Drawing for the job (mm, zero at the part's lowest x, y, z). A direction names the side the tool comes from. Give positions to 0.01 mm unless a question says otherwise; leave off trailing zeros. Write each loop counter-clockwise with the first axis right and the second up, starting at its lowest first coordinate (ties: lowest second). Pieces come first, ordered by that corner, then holes.
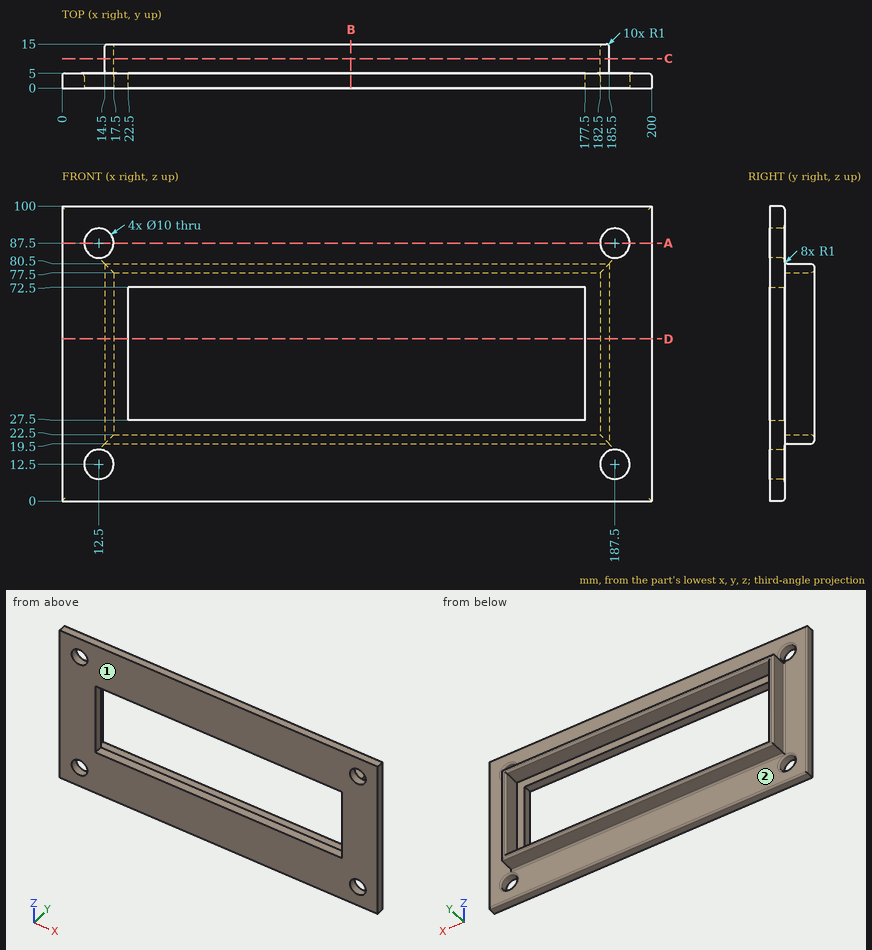
1. Which spindle directions (+Z, -Z, +X, -X, +Y, -Y) get a long thin tool onto all of the face, cutting with end or side? Do the marked faces 1 and 2. Say none if no direction does.
Calculated:
face 1: +Z, -Z, +X, -X, -Y
face 2: +Y
2. Slice it at D-D, the plane z = 55. Write the cut outline in (x, y), and give its area (3 significant figures).
Calculated:
outline: (0, 0) - (22.5, 0) - (22.5, 5) - (17.5, 5) - (17.5, 14) arc R1 ccw to (16.5, 15) - (15.5, 15) arc R1 ccw to (14.5, 14) - (14.5, 6) arc R1 cw to (13.5, 5) - (1, 5) arc R1 ccw to (0, 4) - close; (177.5, 0) - (200, 0) - (200, 4) arc R1 ccw to (199, 5) - (186.5, 5) arc R1 cw to (185.5, 6) - (185.5, 14) arc R1 ccw to (184.5, 15) - (183.5, 15) arc R1 ccw to (182.5, 14) - (182.5, 5) - (177.5, 5) - close
area: 284 mm2
3. Pin check, flat tips, straight feed: P1, Ø8, axis at x = 12.5, z = 12.5, coming from the -Y side; P2, Ø4, axis at x = 98, y = 10, coming from the -Z side; P3, Ø5, axis at x = 36, y = 13, coming from the +Z side; P4, Ø1, axis at y = 11.5, z = 44.5, coming from the -X side. Stop position of each tip, or through.
Calculated:
P1: passes through
P2: stops at z = 19.5
P3: stops at z = 80.5
P4: stops at x = 14.5
4. Probe probe 1 along X at (y, z) = (0.95, 12.5); probe 2 along X at (y, z) = (10, 34); probe 3 along Z at (x, y) = (24, 8.25). List the from-to ranges inside material, lowest first.
Calculated:
probe 1: x = 0 to 7.5, 17.5 to 182.5, 192.5 to 200
probe 2: x = 14.5 to 17.5, 182.5 to 185.5
probe 3: z = 19.5 to 22.5, 77.5 to 80.5
5. Slice it at B-B, the plane x = 98. Write the cut outline in (y, z).
Calculated:
outline: (0, 0) - (4, 0) arc R1 ccw to (5, 1) - (5, 18.5) arc R1 cw to (6, 19.5) - (14, 19.5) arc R1 ccw to (15, 20.5) - (15, 21.5) arc R1 ccw to (14, 22.5) - (5, 22.5) - (5, 27.5) - (0, 27.5) - close; (0, 72.5) - (5, 72.5) - (5, 77.5) - (14, 77.5) arc R1 ccw to (15, 78.5) - (15, 79.5) arc R1 ccw to (14, 80.5) - (6, 80.5) arc R1 cw to (5, 81.5) - (5, 99) arc R1 ccw to (4, 100) - (0, 100) - close
6. Slice it at A-A, the plane z = 87.5. Write the cut outline in (x, y).
Calculated:
outline: (0, 0) - (7.5, 0) - (7.5, 4) arc R1 ccw to (6.5, 5) - (1, 5) arc R1 ccw to (0, 4) - close; (17.5, 0) - (182.5, 0) - (182.5, 4) arc R1 ccw to (181.5, 5) - (18.5, 5) arc R1 ccw to (17.5, 4) - close; (192.5, 0) - (200, 0) - (200, 4) arc R1 ccw to (199, 5) - (193.5, 5) arc R1 ccw to (192.5, 4) - close
7. Slice it at C-C, the plane y = 10. Write the cut outline in (x, z).
Calculated:
outline: (14.5, 19.5) - (185.5, 19.5) - (185.5, 80.5) - (14.5, 80.5) - close; hole (17.5, 22.5) - (182.5, 22.5) - (182.5, 77.5) - (17.5, 77.5) - close
